Source: three-view drawing plus pictorial views. Frame: mm from the lowest corner of the part. Give positions to 0.01 mm unless a question says otherwise; leave off trailing zeros. Order: outer loops, then holes, each group sorted by start corner. A loop starts at its lowest first (then second) coordinate and runs counter-clockwise, first axis right, second up. Notation, with made-up numbers: (-3.75, -34) -> (13.25, -34) arc R25 ccw to (13.25, -2) -> close; hole circle Ø11 at (57.5, -5). An arc over 180 degrees is marked (long way). Answer in a Markdown table with one row per item. Add a question column.
Q1. Line query: line 1 along Y through (x, z) = (14.25, 594) (1 decimal); line 2 along X through (y, z) = (71, 532.5) (1 decimal); line 3 along Y through (x, z) = (18.25, 129.5). Output: solid intervals per line, ascending. Write a range as from..to.
Q2. Cut plane C-C on y = 76.5. Return the cut outline in (x, z) (1 decimal).
Q3. Cut plane A-A on x = 13. Return the cut outline in (y, z) (1 decimal), and give its area (3 significant figures).
Q4. Contact query for flat-ended pins moving along their axis: P1, Ø11.5, axis at y = 88.5, z = 375.5, coming from the +X side (1 decimal); P2, Ø2, axis at x = 12.5, y = 83.5, coming from the +Z side; P3, Ø5, axis at x = 13, z = 403, coming from the +Y side. Output: stop coordinate, or through.
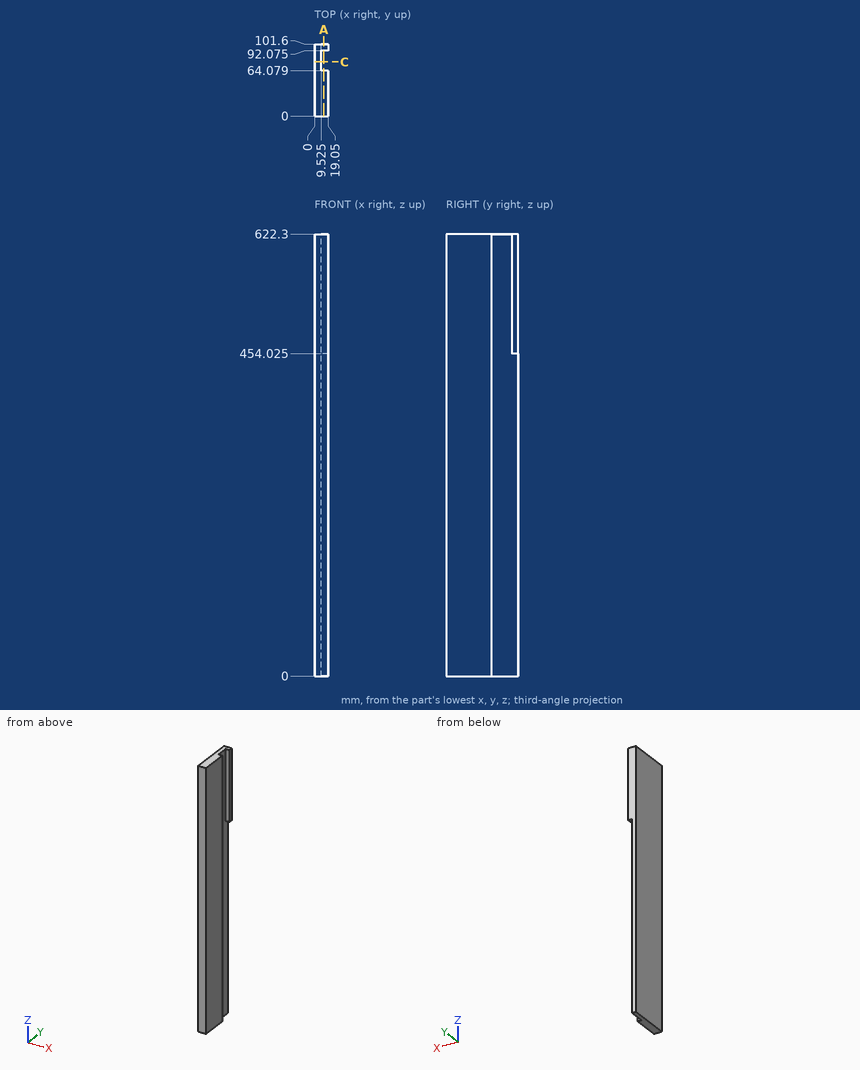
Completed:
| question | item | result |
|---|---|---|
| 1 | line 1 | y = 0..64.1, 92.1..101.6 |
| 1 | line 2 | x = 0..9.5 |
| 1 | line 3 | y = 0..64.08 |
| 2 | outline | (0, 0) -> (9.5, 0) -> (9.5, 622.3) -> (0, 622.3) -> close |
| 3 | outline | (0, 0) -> (64.1, 0) -> (64.1, 622.3) -> (0, 622.3) -> close; (92.1, 454) -> (101.6, 454) -> (101.6, 622.3) -> (92.1, 622.3) -> close |
| 3 | area | 41,500 mm² |
| 4 | P1 | stops at x = 9.5 |
| 4 | P2 | passes through |
| 4 | P3 | stops at y = 64.08 |
